Geometry check sheet. Reference: the model listing, model coordinates, mm. A direction names the side the tool comes from. Round coordinates to 2 decimals unless told otherwise and drop trailing zeros. Write each loop counter-clockwise with the first axis right and the second up, starting at its lowest first coordinate (ties: lowest second). Pieces come first, ordered by that corner, then holes.
Item 1: Depth check by flat-ended pin: P1, Ø1.5, axis at x = -66.5, y = 1, coming from the +Z side; P2, Ø12, axis at x = 49, z = 20, coming from the -Y side; P3, Ø1.5, axis at x = 86.5, y = 2, coming from the +Z side; P4, Ø0.9, axis at y = 2, z = 51.5, coming from the -X side. Enter the tip coordinate at first touch or a pass-through.
Item 2: Cross-section at A-A (x = -30). Enter the section's corners in (y, z).
Item 3: Access from +Z, -Z, +X, -X, +Y, -Y to the whole of each face (thin tool, end or side, straight path). Record for faces 4 (the face through (24, 3, 11)), 5 (the face through (-26.767, 1.479, -3.384)).
Item 4: Cross-section at C-C (y = 1.3). State how many separate pieces and enclosed holes the cut face has, then the cut area to 3 significant figures.
Item 5: Draft check along Z on faces 1 (the face through (24, 0, 11)), 2 (the face through (38, 1, -44)), 3 (the face through (46.18, 1.48, 3.21)). Enter one of: pulls with the +Z half, pulls with the -Z half, needs draft (parallel to the pull), parting line crosses it, or undercut.
Item 6: Cross-section at D-D (x = -66). Enter the section's corners in (y, z), then the cut area to 3 significant figures.
Item 7: Cross-section at B-B (z = -14.5). Enter the section's corners in (x, y), then the cut area to 3 significant figures.
Item 8: Scan lines: probe 1 along X at (y, z) = (2.3, -29.5); probe 2 along X at (y, z) = (2.3, -14.5); probe 3 along Z at (x, y) = (-73, 0.75). Record each from-to range of solid material in increasing order.
Autodesk Inventor part; units mm, degrees
ref_plane "YZ Plane" through (0, 0, 0) normal (1, 0, 0) x (0, 1, 0)
ref_plane "XZ Plane" through (0, 0, 0) normal (0, 1, 0) x (-1, 0, 0)
ref_plane "XY Plane" through (0, 0, 0) normal (0, 0, 1) x (1, 0, 0)
sketch "Sketch2" plane through (0, 0, 0) normal (0, 1, 0) x (-1, 0, 0)
  line L0 (70, -18) -> (60, -18)
  line L1 (60, -18) -> (60, -12)
  line L2 (70, -12) -> (70, -18)
  line L3 (-70, -18.0006) -> (-60, -18.0006)
  line L4 (-60, -18.0006) -> (-60, -12.0003)
  line L5 (-70, -12.0003) -> (-70, -18.0006)
  line L6 (3, 70) -> (-3, 70)
  line L7 (-3, 70) -> (-3, 80)
  line L8 (-3, 80) -> (3, 80)
  line L9 (3, 80) -> (3, 70)
  line L10 (3, 45) -> (-3, 45)
  line L11 (-3, 45) -> (-3, 55)
  line L12 (-3, 55) -> (3, 55)
  line L13 (3, 55) -> (3, 45)
  line L14 (100, -65) -> (-100, -65)
  line L15 (-12.5, 85) -> (12.5, 85)
  line L16 (12.5, 85) -> (35.9015, 46.7742)
  line L17 (-100, -12.0003) -> (-70, -12.0003)
  line L18 (-55.4919, -12.0003) -> (-60, -12.0003)
  line L19 (55.4917, -12) -> (60, -12)
  line L20 (70, -12) -> (100, -12)
  line L21 (-100, -65) -> (-100, -12.0003)
  line L22 (100, -65) -> (100, -12)
  line L23 (35, -45) -> (-35, -45)
  line L24 (-40, -40) -> (-40, -26.409)
  line L25 (-39.2644, -23.7983) -> (-13.9141, 17.6106)
  line L26 (-9.6497, 20) -> (9.6497, 20)
  line L27 (40, -40) -> (40, -26.409)
  line L28 (39.2644, -23.7983) -> (13.9141, 17.6106)
  arc A0 (-40, -40) -> (-35, -45) centre (-35, -40) ccw
  arc A1 (-39.2644, -23.7983) -> (-40, -26.409) centre (-35, -26.409) ccw
  arc A2 (-9.6497, 20) -> (-13.9141, 17.6106) centre (-9.6497, 15) ccw
  arc A3 (13.9141, 17.6106) -> (9.6497, 20) centre (9.6497, 15) ccw
  arc A4 (40, -26.409) -> (39.2644, -23.7983) centre (35, -26.409) ccw
  arc A5 (35, -45) -> (40, -40) centre (35, -40) ccw
  line L29 (55.4917, -12) -> (35.9015, 20)
  line L30 (35.9015, 20) -> (35.9015, 46.7742)
  line L31 (-55.4919, -12.0003) -> (-35.9015, 20)
  line L32 (-35.9015, 20) -> (-35.9015, 46.7742)
  line L33 (-35.9015, 46.7742) -> (-12.5, 85)
  line L34 (0, -65) -> (0, 85) construction
  point P0 (0, 0)
  point P1 (0, 80)
  point P2 (0, 45)
  point P3 (0, 55)
  point P4 (0, 0)
  point P5 (0, 0)
  point P6 (-70, -15.4178)
  point P7 (75.3708, -12)
  point P8 (0, 0)
  point P9 (-40, -45)
  point P10 (40, -45)
  point P11 (-40, -25)
  point P12 (-12.4513, 20)
  point P13 (12.4513, 20)
  point P14 (40, -25)
  point P15 (0, 20)
  point P16 (0, -45)
  point P17 (0, 85)
  dimension "d65" = 200
  dimension "d115" = 10
  dimension "d116" = 6
  dimension "d118" = 10
  dimension "d119" = 6
  dimension "d120" = 15
  dimension "d147" = 65
  dimension "d173" = 25
  dimension "d187" = 100
  dimension "d191" = 30
  dimension "d192" = 30
  dimension "d194" = 6.0003
  dimension "d195" = 6
  dimension "d196" = 10
  dimension "d197" = 10
  dimension "d198" = 52.9997
  dimension "d199" = 53
  dimension "d204" = 150
  dimension "d213" = 20
  dimension "d214" = 20
  dimension "d218" = 65
  dimension "d219" = 40
  dimension "d220" = 5
  dimension "d233" = 148.525
  dimension "d235" = 5
  dimension "d236" = 20
extrude "Extrusion11" add sketch "Sketch2" along normal blind 3
sketch "Sketch4" plane through (0, 3, 0) normal (0, 1, 0) x (1, 0, 0)
  line L0 (-51, 38) -> (-45, 38)
  line L1 (-45, 38) -> (-45, 28)
  line L2 (-45, 28) -> (-51, 28)
  line L3 (-51, 28) -> (-51, 38)
  line L4 (100, 65) -> (-100, 65)
  line L5 (-40, 40) -> (-40, 26.409)
  line L6 (45, 38) -> (51, 38)
  line L7 (51, 38) -> (51, 28)
  line L8 (51, 28) -> (45, 28)
  line L9 (45, 28) -> (45, 38)
  line L10 (40, 40) -> (40, 26.409)
  point P0 (0, 0)
  dimension "d237" = 6
  dimension "d238" = 27
  dimension "d239" = 10
  dimension "d240" = 5
  dimension "d241" = 6
  dimension "d242" = 10
  dimension "d243" = 5
  dimension "d244" = 27
extrude "Extrusion13" cut sketch "Sketch4" against normal through all
fillet "Fillet1" radius 15 6 edges at (12.5, 1.5, 85) (-12.5, 1.5, 85) (-35.9015, 1.5, 46.7742) (35.9015, 1.5, 46.7742) (35.9015, 1.5, 20) (-35.9015, 1.5, 20)
fillet "Fillet2" radius 5 2 edges at (55.4919, 1.5, -12.0003) (-55.4917, 1.5, -12)
properties part number "Top Plate 27100914"
Resolved:
1. P1: stops at z = -18
1. P2: passes through
1. P3: stops at z = -12
1. P4: stops at x = -33.28
2. outline: (0, -65) - (3, -65) - (3, -45) - (0, -45) - close; (0, -8.67) - (3, -8.67) - (3, 56.41) - (0, 56.41) - close
3. face 4: +Z, -Z, +X, -X, +Y
3. face 5: +Y, -Y
4. separate pieces: 1
4. enclosed holes: 5
4. area: 13,000 mm2
5. face 1: needs draft
5. face 2: undercut
5. face 3: pulls with the +Z half
6. outline: (0, -65) - (3, -65) - (3, -18) - (0, -18) - close
6. area: 141 mm2
7. outline: (-100, 0) - (-70, 0) - (-70, 3) - (-100, 3) - close; (-60, 0) - (-33.57, 0) - (-33.57, 3) - (-60, 3) - close; (33.57, 0) - (60, 0) - (60, 3) - (33.57, 3) - close; (70, 0) - (100, 0) - (100, 3) - (70, 3) - close
7. area: 339 mm2
8. probe 1: x = -100 to -51, -45 to -40, 40 to 45, 51 to 100
8. probe 2: x = -100 to -70, -60 to -33.57, 33.57 to 60, 70 to 100
8. probe 3: z = -65 to -12
